Geometry: final body of the model. Coordinates: model frame, mm. Face numbers are marked on the shaded views. A direction names the side the tool comes from. Coordinates: 2 decimals unless noted, no trailing zeros. Write each loop counter-clockwise with the first axis right and the second up, starting at its lowest first coordinate (ties: lowest second). Pieces come first, ordered by that corner, then holes. Notation, with made-up numbers: (39, 1) - (50, 1) arc R21 ccw to (50, 6) - close; hole circle Ø3 at (6.5, 71.5). An arc over 180 degrees is marked (long way). Put each result on its own line as item: value.
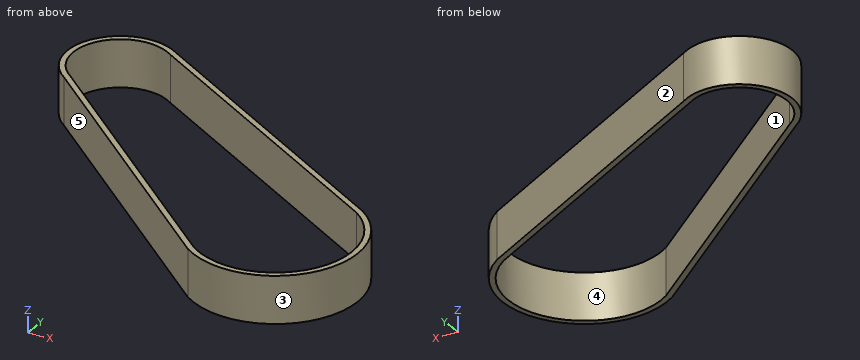
```python
from build123d import *

# Parameters (mm, degrees)
BOSS_EXTRU_1_DEPTH = 8


with BuildPart() as part:
    # Esquisse1 → Boss.-Extru.1 (new body)
    with BuildSketch(Plane.XY):
        with BuildLine():
            Line((8.113333009, 11.409374544), (-39.892627503, 39.410448447))
            ThreePointArc((-39.892627503, 39.410448447), (-52.372722195, 37.161682616), (-50.215714077, 24.665402079))
            Line((-50.215714077, 24.665402079), (-8.113333009, -11.409374544))
            ThreePointArc((-8.113333009, -11.409374544), (11.409374544, -8.113333009), (8.113333009, 11.409374544))
        make_face()
        with BuildLine():
            ThreePointArc((-49.636190291, 25.480357403), (-51.519642597, 36.636190291), (-40.363809709, 38.519642597))
            Line((-40.363809709, 38.519642597), (7.533809223, 10.594419219))
            ThreePointArc((7.533809223, 10.594419219), (10.594419219, -7.533809223), (-7.533809223, -10.594419219))
            Line((-7.533809223, -10.594419219), (-49.636190291, 25.480357403))
        make_face(mode=Mode.SUBTRACT)
    extrude(amount=BOSS_EXTRU_1_DEPTH)


solid = part.part
```
1. Set-up query: the marked faces 1 and 2. Return all of +Z, -Z, +X, -X, +Y, -Y with unobstructed straight access to the full face (end or side cutting, diameter ignored); none if empty.
Answer below:
face 1: +Z, -Z
face 2: +Z, -Z, +X, +Y
2. Ray query, probe 1 along Y at (x, z) = (2, 3.5); probe 2 along Y at (x, z) = (-6.5, 5.5); probe 3 along X at (y, z) = (-5, 3). Return the intervals inside material, ascending. Write a range as from..to.
Answer below:
probe 1: y = -13.86..-12.85, 13.82..14.98
probe 2: y = -12.4..-11.26, 18.78..19.93
probe 3: x = -15.59..-14.06, 12..13.08
3. Pin query (flat end, axial travel): pin 1 Ø1 at (y, z) = (11, 1.5) entering from +X; pin 2 Ø4 at (y, z) = (10.5, 6.5) entering from -X; pin 3 Ø3 at (x, z) = (-3.5, 6) entering from -Y. Return the tip coordinate at first contact, or that it passes through.
Answer below:
pin 1: stops at x = 9.26
pin 2: stops at x = -36.02
pin 3: stops at y = -13.86
4. Section query B-B (x = 0). Return loops of the section in (y, z), then the cut area to 3 significant figures.
Answer below:
outline: (-14, 0) - (-13, 0) - (-13, 8) - (-14, 8) - close; (14.99, 0) - (16.14, 0) - (16.14, 8) - (14.99, 8) - close
area: 17.2 mm²
5. Section query A-A (y = 3.5). Return loops of the section in (x, z).
Answer below:
outline: (-25.51, 0) - (-23.98, 0) - (-23.98, 8) - (-25.51, 8) - close; (12.52, 0) - (13.56, 0) - (13.56, 8) - (12.52, 8) - close
6. Mould query, pull axis Y, two halves, no side actions, for the marked faces 3, 4 and 5. Classes: +Y half, -Y half, draft (parallel to the pull), parting line (faces both ways), or undercut.
Answer below:
face 3: parting line
face 4: undercut
face 5: -Y half
